from build123d import *

# Parameters (mm, degrees)
F0_W      = 114.3
F0_H      = 114.3
F0_W_2    = 101.6
F0_H_2    = 101.6
F1_DEPTH  = 12.7
F2_W      = 114.3
F2_H      = 114.3
F3_DEPTH  = 0.6096
F4_W      = 20.8788
F4_H      = 3.302
F5_DEPTH  = 17.78
F6_R      = 6.6294
F8_DEPTH  = 6.35
F9_R      = 6.6294
F10_R     = 4.445
F11_DEPTH = 1.27
F12_R     = 4.445
F13_DEPTH = 1.27
F14_SIZE  = 1.26999
F15_W     = 15.24
F15_H     = 8.89
F16_DEPTH = 1.5875
F17_R     = 4.44499
F18_R     = 3.175
F19_DEPTH = 25.4


# Not quite as in the source:
# - a fillet or chamfer is up to 0.001 mm smaller than in the source, because OpenCascade refuses the exact size
# - a pattern or mirror of a feature is missing from the dataset's text; its kind, count and spacing are read off the source's solid


with BuildPart() as f1:
    # F0 (on Right) → F1 (new body)
    with BuildSketch(Plane.YZ):
        Rectangle(F0_W, F0_H)
        Rectangle(F0_W_2, F0_H_2, mode=Mode.SUBTRACT)
    extrude(amount=F1_DEPTH)

    # F2 (on Right) → F3 (join)
    with BuildSketch(Plane.YZ):
        Rectangle(F2_W, F2_H)
    extrude(amount=-F3_DEPTH)

    # F4 (on face) → F5 (join)
    with BuildSketch(Plane.XY.offset(57.15)):
        with Locations((15.5194, -45.974)):
            Rectangle(F4_W, F4_H)
    f5 = extrude(amount=F5_DEPTH)

    # F5_copies: F5 across plane
    add(f5.mirror(Plane.ZX))

    # F6
    f6_edges = [f1.edges().sort_by_distance(p)[0] for p in [
        (25.9588, -45.974, 74.93),
    ]]
    fillet(f6_edges, radius=F6_R)

    # F7 (on face) → F8 (cut)
    with BuildSketch(Plane.XZ.offset(47.625)):
        with BuildLine():
            ThreePointArc((19.3294, 74.93), (25.9588, 68.3006), (19.3294, 61.6712))
            Line((19.3294, 61.6712), (12.7, 61.6712))
            Line((12.7, 61.6712), (12.7, 57.15))
            Line((12.7, 57.15), (28.7029210806, 51.0326394975))
            Line((28.7029210806, 51.0326394975), (31.0219925225, 81.4440133214))
            Line((31.0219925225, 81.4440133214), (19.3294, 74.93))
        make_face()
    f8 = extrude(amount=-F8_DEPTH, mode=Mode.SUBTRACT)

    # F8_copies: F8 across plane
    add(f8.mirror(Plane.ZX), mode=Mode.SUBTRACT)

    # F9
    f9_edges = [f1.edges().sort_by_distance(p)[0] for p in [
        (5.08, -45.974, 74.93),
        (5.08, 45.974, 74.93),
    ]]
    fillet(f9_edges, radius=F9_R)

    # F10 (on face) → F11 (join)
    with BuildSketch(Plane.XZ.offset(47.625)):
        with Locations((19.3294, 68.3006)):
            Circle(F10_R)
    f11 = extrude(amount=F11_DEPTH)

    # F11_copies: F11 across plane
    add(f11.mirror(Plane.ZX))

    # F12 (on face) → F13 (join)
    with BuildSketch(Plane(origin=(0, -44.323, 0), x_dir=(-1, 0, 0), z_dir=(0, 1, 0))):
        with Locations((-19.3294, 68.3006)):
            Circle(F12_R)
    f13 = extrude(amount=F13_DEPTH)

    # F13_copies: F13 across plane
    add(f13.mirror(Plane.ZX))

    # F14 (size 1.27 in the source; OpenCascade refuses exactly that, so slightly less here)
    f14_edges = [f1.edges().sort_by_distance(p)[0] for p in [
        (14.8844, -48.895, 68.3006),
        (23.7744, -43.053, 68.3006),
        (14.8844, 48.895, 68.3006),
        (23.7744, 43.053, 68.3006),
    ]]
    chamfer(f14_edges, length=F14_SIZE)

    # F15 (on Front) → F16 (join, symmetric)
    with BuildSketch(Plane.XZ):
        with Locations((13.97, -61.595)):
            Rectangle(F15_W, F15_H)
    extrude(amount=F16_DEPTH, both=True)

    # F17 (radius 4.445 in the source; OpenCascade refuses exactly that, so slightly less here)
    f17_edges = [f1.edges().sort_by_distance(p)[0] for p in [
        (21.59, 0, -57.15),
        (21.59, 0, -66.04),
        (6.35, 0, -66.04),
    ]]
    fillet(f17_edges, radius=F17_R)

    # F18 (on face) → F19 (cut)
    with BuildSketch(Plane(origin=(0, 1.5875, 0), x_dir=(-1, 0, 0), z_dir=(0, 1, 0))):
        with Locations((-17.145, -61.595)):
            Circle(F18_R)
    extrude(amount=-F19_DEPTH, mode=Mode.SUBTRACT)


solid = f1.part
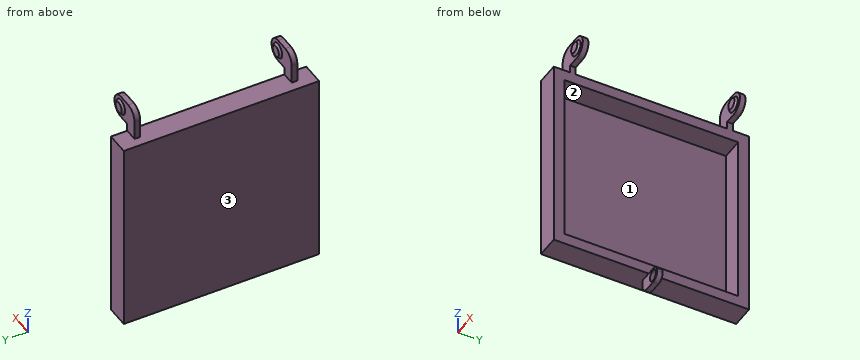
Read the model definition and answer for the solid it produces. Units are mm, in the model's axes. Face numbers are marked on the shaded views. Round coordinates to 2 decimals unless told otherwise and drop trailing zeros. Order: outer loops, then holes, each group sorted by start corner. A loop starts at its lowest first (then second) coordinate and runs counter-clockwise, first axis right, second up.
1) The mould has two halves that part along Y. Classify the marked faces 1, 2 and 3: released by +Y, released by -Y, zero draft, split by the parting line, or undercut.
2) Straight lines are drawn through the part: L1, parallel to Y at x = 5.25, z = 23.5; L2, parallel to Y at x = 23.75, z = 69.5 (3 decimals). For each, find the intervals that lie inside material, in ascending order.
3) The part is cut by section D-D on y = -46. Write down the section's boundary in (x, z), plus the area to 3 significant figures.
4) Flat-ended cylindrical pins translate along their axes: pin 1 (1.5 mm diameter, centred on y = -41, z = 18, fed in from +X); pin 2 (6.5 mm diameter, centred on x = 9, y = 23, fed in from +Z); pin 3 (6.5 mm diameter, centred on x = 6, y = 12.5, fed in from -Z); pin 4 (4 mm diameter, centred on x = 16.5, z = 59.5, fed in from +Y). Find the tip coordinate at first contact, or state that the pin passes through.
5) The part is cut by section A-A on z = -6. Write down the section's boundary in (x, y).
Resolved:
1. face 1: undercut
1. face 2: undercut
1. face 3: zero draft
2. L1: y = -57.15 to -50.8, 50.8 to 57.15
2. L2: y = -47.625 to -44.323, 44.323 to 47.625
3. outline: (-0.61, -57.15) - (12.7, -57.15) - (12.7, -50.8) - (0, -50.8) - (0, 50.8) - (12.7, 50.8) - (12.7, 61.67) - (19.33, 61.67) arc R6.63 ccw to (19.33, 74.93) - (11.71, 74.93) arc R6.63 ccw to (5.08, 68.3) - (5.08, 57.15) - (-0.61, 57.15) - close
3. area: 514 mm2
4. pin 1: stops at x = 0
4. pin 2: stops at z = 57.15
4. pin 3: stops at z = -57.15
4. pin 4: passes through
5. outline: (-0.61, -57.15) - (12.7, -57.15) - (12.7, -50.8) - (0, -50.8) - (0, 50.8) - (12.7, 50.8) - (12.7, 57.15) - (-0.61, 57.15) - close
